from build123d import *

# Parameters (mm, degrees)
F0_W     = 3
F0_H     = 9.1476
F1_DEPTH = 60
F2_R     = 2
F3_R     = 1


with BuildPart() as f1:
    # F0 (on Top) → F1 (new body)
    with BuildSketch(Plane.XY):
        with Locations((-23.505458, -12.97862)):
            Rectangle(F0_W, F0_H)
        Polygon((76.056968, 12.94758), (-22.005458, 12.94758), (-22.005458, -8.40482), (-22.005458, -17.55242), (-17.005458, -17.55242), (-17.005458, -14.55242), (-19.974245, -14.55242), (-19.974245, -12.35242), (-17.005458, -12.35242), (-17.005458, 7.983583), (71.056968, 7.983583), (71.056968, -12.35242), (74.025755, -12.35242), (74.025755, -14.55242), (71.056968, -14.55242), (71.056968, -17.55242), (76.056968, -17.55242), (76.056968, -8.40482), align=None)
        with Locations((77.556968, -12.97862)):
            Rectangle(F0_W, F0_H)
    extrude(amount=F1_DEPTH)

    # F2
    f2_edges = [f1.edges().sort_by_distance(p)[0] for p in [
        (-22.005458, 12.94758, 30),
        (76.056968, 12.94758, 30),
        (-25.005458, -8.40482, 30),
        (-25.005458, -17.55242, 30),
        (79.056968, -8.40482, 30),
        (79.056968, -17.55242, 30),
        (-17.005458, 7.983583, 30),
        (71.056968, 7.983583, 30),
    ]]
    fillet(f2_edges, radius=F2_R)

    # F3
    f3_edges = [f1.edges().sort_by_distance(p)[0] for p in [
        (-18.489851, -14.55242, 0),
        (-18.489851, -12.35242, 0),
        (-19.974245, -13.45242, 0),
        (-18.489851, -12.35242, 60),
        (-19.974245, -13.45242, 60),
        (-18.489851, -14.55242, 60),
        (72.541362, -14.55242, 0),
        (-25.005458, -12.97862, 0),
        (-24.419671, -8.990607, 0),
        (-24.419671, -16.966634, 0),
        (-22.505458, -8.40482, 0),
        (-20.005458, -17.55242, 0),
        (-22.005458, 1.27138, 0),
        (-17.005458, -16.05242, 0),
        (-21.419671, 12.361793, 0),
        (27.025755, 12.94758, 0),
        (75.471182, 12.361793, 0),
        (76.056968, 1.27138, 0),
        (-17.005458, -3.184419, 0),
        (76.556968, -8.40482, 0),
        (-16.419671, 7.397797, 0),
        (78.471182, -8.990607, 0),
        (27.025755, 7.983583, 0),
        (79.056968, -12.97862, 0),
        (70.471182, 7.397797, 0),
        (78.471182, -16.966634, 0),
        (71.056968, -3.184419, 0),
        (74.056968, -17.55242, 0),
        (72.541362, -12.35242, 0),
        (71.056968, -16.05242, 0),
        (74.025755, -13.45242, 0),
        (72.541362, -14.55242, 60),
        (74.025755, -13.45242, 60),
        (72.541362, -12.35242, 60),
    ]]
    fillet(f3_edges, radius=F3_R)


solid = f1.part
Input: part model. Units: mm. Frame: model coordinates. A direction names the side the tool comes from. Give positions to 0.01 mm unless a question says otherwise; leave off trailing zeros. Loops run counter-clockwise (first coordinate to the right, second up) from the corner with the lowest first, then second, coordinate; pieces in that order, holes last. Notation, with made-up numbers: M 59.25,-26 L 103.25,-26 A23 ccw 103.25,12 Z; hole C -7.75,34 d4. An arc over 180 degrees is marked long. Use one line per item in the form item = value.
1. Section query C-C, the plane z = 13. Return the cut outline in (x, y).
Numbers:
outline = M -25.01,-15.55 A2 ccw -23.01,-17.55 L -17.01,-17.55 L -17.01,-14.55 L -19.97,-14.55 L -19.97,-12.35 L -17.01,-12.35 L -17.01,5.98 A2 cw -15.01,7.98 L 69.06,7.98 A2 cw 71.06,5.98 L 71.06,-12.35 L 74.03,-12.35 L 74.03,-14.55 L 71.06,-14.55 L 71.06,-17.55 L 77.06,-17.55 A2 ccw 79.06,-15.55 L 79.06,-10.4 A2 ccw 77.06,-8.4 L 76.06,-8.4 L 76.06,10.95 A2 ccw 74.06,12.95 L -20.01,12.95 A2 ccw -22.01,10.95 L -22.01,-8.4 L -23.01,-8.4 A2 ccw -25.01,-10.4 Z
2. Line query: L1, parallel to X at y = 0, z = 43; L2, parallel to X at y = 8.5, z = 8; L3, parallel to X at y = -13, z = 27.5. Output: solid intervals per line, ascending.
Numbers:
L1 = -22.01 to -17.01, 71.06 to 76.06
L2 = -22.01 to 76.06
L3 = -25.01 to -19.97, 74.03 to 79.06
3. Section query A-A, the plane y = 0. Return the cut outline in (x, z).
Numbers:
outline = M -22.01,1 A1 ccw -21.01,0 L -18.01,0 A1 ccw -17.01,1 L -17.01,60 L -22.01,60 Z; M 71.06,1 A1 ccw 72.06,0 L 75.06,0 A1 ccw 76.06,1 L 76.06,60 L 71.06,60 Z
4. Section query B-B, the plane x = 25.5. Return the cut outline in (y, z), and give its area (3 significant figures).
Numbers:
outline = M 7.98,1 A1 ccw 8.98,0 L 11.95,0 A1 ccw 12.95,1 L 12.95,60 L 7.98,60 Z
area = 297 mm²
5. Pull-direction query (X, two-part tool) for faces 1 (the face through (-21.4, 12.38, 30.91)), 2 (the face through (79.057, -13, 30)), 3 (the face through (26, 11, 60)), 4 (the face through (74.026, -13, 30)); classes: released by +X, released by -X, zero draft, split by the parting line, or undercut.
Numbers:
face_1 = released by -X
face_2 = released by +X
face_3 = zero draft
face_4 = undercut
6. First-contact query: pin 1 (1 mm diameter, centred on y = -3, z = 53, fed in from +X); pin 2 (14.5 mm diameter, centred on y = -2, z = 44.5, fed in from +X); pin 3 (4 mm diameter, centred on x = 30.5, z = 35, fed in from -Y); pin 4 (6 mm diameter, centred on x = 53.5, y = 3.5, fed in from +Z). Flat tips, straight axial feed; report the tip coordinate or a pass-through.
Numbers:
pin_1 = 76.06
pin_2 = 78.69
pin_3 = 7.98
pin_4 = through
7. Reachability of faces 5 (the face through (-18, -14.552, 30)), 6 (the face through (76.057, 1, 30)), 7 (the face through (70.46, 7.41, 30.91)) from +Z, -Z, +X, -X, +Y, -Y: full face, straight path, thin tool, end or side. Return the list, or none.
Numbers:
face_5 = +Z, -Z
face_6 = +Z, -Z, +X, +Y
face_7 = +Z, -Z, -Y
